Here's how the part is built. I have some questions about the finished solid (model axes, mm). Face numbers are marked on the shaded views. A direction names the side the tool comes from. Coordinates: 2 decimals unless noted, no trailing zeros. Order: outer loops, then holes, each group sorted by start corner. A loop starts at its lowest first (then second) coordinate and runs counter-clockwise, first axis right, second up. Notation, with made-up numbers: (64, -0.5) - (89, -0.5) arc R20 cw to (89, 36.5) - close; hole circle Ø11 at (89.25, 55.25). An arc over 180 degrees is marked (long way). Answer in a Markdown table with one row per item. Add a question column.
Item 1: I want a section at A-A (x = -12). Please give me the cut outline in (y, z) (3 decimals).
Item 2: I want a section at C-C (y = 5.5). Please give me the cut outline in (x, z) (3 decimals).
Item 3: Thinking about a two-plate mould opening in X: for the marked faces 5, 6 and 7, which applies, +X half, -X half, draft (parallel to the pull), parting line (faces both ways), or undercut?
Item 4: On a 3-axis mill with a long thin cutter (end or side, diameter ignored), from which of +Z, -Z, +X, -X, +Y, -Y can I reach the whole of each face in a straight line? I mean the marked faces 1, 2, 3 and 4. Say none if no direction works.
Item 5: I want a section at B-B (z = -1.05). Please give me the cut outline in (x, y), plus the area to 3 significant figures.
Item 6: Will these pins go through, and if not, where does the flat tip stop? pin 1 Ø0.6 at (x, z) = (-10.5, 1.5) entering from +Y; pin 2 Ø3 at (x, y) = (-10.5, 1) entering from +Z; pin 3 Ø2 at (x, y) = (-12, -2) entering from -Z; pin 4 Ø1.4 at (x, y) = (11.5, 2) entering from -Z (3 decimals).
Item 7: If I drill on line 1 along Z through (x, y) = (-12, -3.75) (3 decimals); line 2 along X through (y, z) = (3, 0.85); line 3 along Z through (x, y) = (10.5, 5.5) (3 decimals), over which ranges is the centre line in solid material (lowest first)? Write a range as from..to.
Item 8: I want a section at D-D (y = -5). Please give me the cut outline in (x, z) (3 decimals), plus the area to 3 significant figures.
```python
from build123d import *

# Parameters (mm, degrees)
SKETCH1_W           = 22
SKETCH1_H           = 14
SKETCH1_R           = 1.275
BOSS_EXTRUDE1_DEPTH = 0.475
SKETCH2_W           = 2.6
SKETCH2_H           = 13.1
BOSS_EXTRUDE2_DEPTH = 1.855
SKETCH3_W           = 1.25
SKETCH3_H           = 12.5
BOSS_EXTRUDE3_DEPTH = 2.5
SKETCH4_W           = 4.3
SKETCH4_H           = 4.6
BOSS_EXTRUDE4_DEPTH = 2


with BuildPart() as part:
    # Sketch1 → Boss-Extrude1 (new body, symmetric)
    with BuildSketch(Plane.XY):
        Rectangle(SKETCH1_W, SKETCH1_H)
        with Locations((8.225, -4.225)):
            Circle(SKETCH1_R, mode=Mode.SUBTRACT)
    extrude(amount=BOSS_EXTRUDE1_DEPTH, both=True)

    # Sketch2 → Boss-Extrude2 (add)
    with BuildSketch(Plane.XY.offset(0.475)):
        with Locations((-9.81, 0)):
            Rectangle(SKETCH2_W, SKETCH2_H)
    boss_extrude2 = extrude(amount=BOSS_EXTRUDE2_DEPTH)

    # Mirror1: Boss-Extrude2 across plane
    add(boss_extrude2.mirror(Plane.XY))

    # Sketch3 → Boss-Extrude3 (add)
    with BuildSketch(Plane.ZY.offset(11.11)):
        with Locations((-1.4, 0)):
            Rectangle(SKETCH3_W, SKETCH3_H)
    boss_extrude3 = extrude(amount=BOSS_EXTRUDE3_DEPTH)

    # Mirror2: Boss-Extrude3 across plane
    add(boss_extrude3.mirror(Plane.XY))

    # Sketch4 → Boss-Extrude4 (add)
    with BuildSketch(Plane.XY.offset(0.475)):
        with Locations((10.1, 1.7)):
            Rectangle(SKETCH4_W, SKETCH4_H)
    extrude(amount=BOSS_EXTRUDE4_DEPTH)


solid = part.part
```
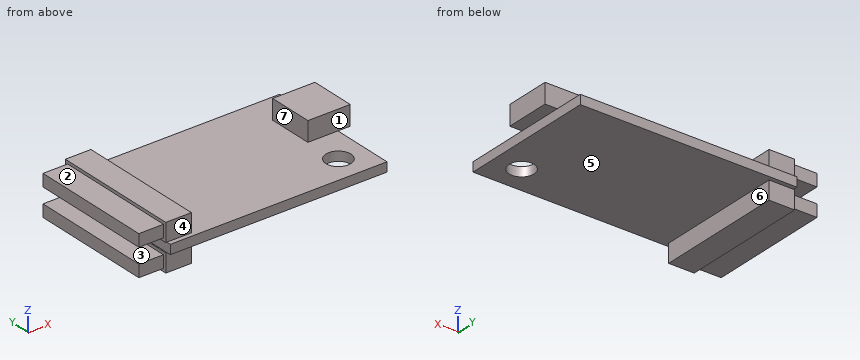
Values follow:
| question | item | result |
|---|---|---|
| 1 | outline | (-6.25, -2.025) - (6.25, -2.025) - (6.25, -0.775) - (-6.25, -0.775) - close; (-6.25, 0.775) - (6.25, 0.775) - (6.25, 2.025) - (-6.25, 2.025) - close |
| 2 | outline | (-13.61, -2.025) - (-11.11, -2.025) - (-11.11, -2.33) - (-8.51, -2.33) - (-8.51, -0.475) - (11, -0.475) - (11, 0.475) - (-8.51, 0.475) - (-8.51, 2.33) - (-11.11, 2.33) - (-11.11, 2.025) - (-13.61, 2.025) - (-13.61, 0.775) - (-11.11, 0.775) - (-11.11, 0.475) - (-11, 0.475) - (-11, -0.475) - (-11.11, -0.475) - (-11.11, -0.775) - (-13.61, -0.775) - close |
| 3 | face 5 | draft |
| 3 | face 6 | +X half |
| 3 | face 7 | undercut |
| 4 | face 1 | +Z, +X, -Y |
| 4 | face 2 | +Z, -X, +Y, -Y |
| 4 | face 3 | -X, +Y, -Y |
| 4 | face 4 | +Z, +X, -X, -Y |
| 5 | outline | (-13.61, -6.25) - (-11.11, -6.25) - (-11.11, -6.55) - (-8.51, -6.55) - (-8.51, 6.55) - (-11.11, 6.55) - (-11.11, 6.25) - (-13.61, 6.25) - close |
| 5 | area | 65.3 mm^2 |
| 6 | pin 1 | stops at y = 6.55 |
| 6 | pin 2 | stops at z = 2.33 |
| 6 | pin 3 | stops at z = -2.33 |
| 6 | pin 4 | stops at z = -0.475 |
| 7 | line 1 | z = -2.025..-0.775, 0.775..2.025 |
| 7 | line 2 | x = -13.61..-8.51, 7.95..12.25 |
| 7 | line 3 | z = -0.475..0.475 |
| 8 | outline | (-13.61, -2.025) - (-11.11, -2.025) - (-11.11, -2.33) - (-8.51, -2.33) - (-8.51, -0.475) - (7.213, -0.475) - (7.213, 0.475) - (-8.51, 0.475) - (-8.51, 2.33) - (-11.11, 2.33) - (-11.11, 2.025) - (-13.61, 2.025) - (-13.61, 0.775) - (-11.11, 0.775) - (-11.11, 0.475) - (-11, 0.475) - (-11, -0.475) - (-11.11, -0.475) - (-11.11, -0.775) - (-13.61, -0.775) - close; (9.237, -0.475) - (11, -0.475) - (11, 0.475) - (9.237, 0.475) - close |
| 8 | area | 34.9 mm^2 |
